Here's how the part is built. I have some questions about the finished solid (model axes, mm). A direction names the side the tool comes from. Coordinates: 2 decimals unless noted, no trailing zeros. Write each loop counter-clockwise with the first axis right and the second up, starting at its lowest first coordinate (ties: lowest second). Pieces come first, ordered by that corner, then holes.
from build123d import *

# Parameters (mm, degrees)
SKETCH3_R                   = 2.5
CUT_EXTRUDE1_DEPTH          = 10
CHAMFER1_SIZE               = 3
M8_TAPPED_HOLE1_D           = 6.8
M8_TAPPED_HOLE1_DEPTH       = 19.75
M8_TAPPED_HOLE1_CSINK_D     = 8.05
M8_TAPPED_HOLE1_CSINK_ANGLE = 90
M8_TAPPED_HOLE1_TIP         = 2.042926105


with BuildPart() as part:
    # Sketch1 → Revolve1 (revolve)
    with BuildSketch(Plane.XY, mode=Mode.PRIVATE) as revolve1_sk:
        Polygon((43, 0), (43, 10), (22.5, 10), (22.5, 20), (8.5, 20), (8.5, 9), (5, 9), (5, 3), (25, 3), (25, 0), align=None)
    revolve(revolve1_sk.sketch.rotate(Axis((0, 0, 0), (0, -1, 0)), 90), axis=Axis((0, 0, 0), (0, -1, 0)))

    # Sketch3 → Cut-Extrude1 (cut)
    with BuildSketch(Plane(origin=(0, 10, 0), x_dir=(1, 0, 0), z_dir=(0, 1, 0))):
        with Locations(Location((34, 0, 0), (0, 0, 270))):
            Circle(SKETCH3_R)
        with Locations(Location((0, -34, 0), (0, 0, 270))):
            Circle(SKETCH3_R)
        with Locations(Location((-34, 0, 0), (0, 0, 270))):
            Circle(SKETCH3_R)
        with Locations(Location((0, 34, 0), (0, 0, 270))):
            Circle(SKETCH3_R)
    extrude(amount=-CUT_EXTRUDE1_DEPTH, mode=Mode.SUBTRACT)

    # Chamfer1
    chamfer1_edges = [part.edges().sort_by_distance(p)[0] for p in [
        (0, 20, -22.5),
    ]]
    chamfer(chamfer1_edges, length=CHAMFER1_SIZE)

    # M8 Tapped Hole1
    with Locations(Plane(origin=(0, 10, -34), x_dir=(0, 0, 1), z_dir=(0, 1, 0))):
        with Locations((0, 0), (34, 34), (68, 0), (34, -34)):
            CounterSinkHole(M8_TAPPED_HOLE1_D / 2, M8_TAPPED_HOLE1_CSINK_D / 2, depth=M8_TAPPED_HOLE1_DEPTH, counter_sink_angle=M8_TAPPED_HOLE1_CSINK_ANGLE)
            with Locations((0, 0, -(M8_TAPPED_HOLE1_DEPTH + M8_TAPPED_HOLE1_TIP / 2))):  # 118° drill point
                Cone(0, M8_TAPPED_HOLE1_D / 2, M8_TAPPED_HOLE1_TIP, mode=Mode.SUBTRACT)


solid = part.part
1. Thinking about a two-plate mould opening in Z: for faces 1 (the face through (-5.901, 19.854, 18.738)), 2 (the face through (4, 9, 4)), 3 (the face through (19, 10, 19)), which applies, pulls with the +Z half, pulls with the -Z half, needs draft (parallel to the pull), parting line crosses it, or undercut?
2. I want a section at D-D (y = 13). List the corners of the cut face in (x, z) for me, then the cut area to 3 significant figures.
3. On a 3-axis mill with a long thin cutter (end or side, diameter ignored), from which of +Z, -Z, +X, -X, +Y, -Y can I reach the whole of each face in a straight line? I mean faces 4 (the face through (-8.428, 14.423, -1.107)), 5 (the face through (-1.3, 4.62, -37.14)), 6 (the face through (-7.509, 1.479, 23.846)). Say none if no direction works.
4. For pin 1 Ø2 at (x, z) = (-16, -15) entering from -Y; pin 2 Ø4 at (y, z) = (11, -17.5) entering from +X; pin 3 Ø22 at (x, z) = (0, 0) entering from +Y; pin 4 Ø8.5 at (x, z) = (-1, 3) entering from +Y, each with a flat end and sliding along its axis, tell me the tip position at first contact or that it passes through.
5. If I drill on line 1 (Y direction, x = -4, z = 35.5); line 2 (Z direction, x = -4, y = 3.5); line 3 (Y direction, x = 8.5, z = -7), over which ranges is the centre line in solid material (lowest first)?
6. I want a section at A-A (x = 0). State how many separate pieces and enclosed holes the cut face has, then the cut area to 3 significant figures.
7. I want a section at B-B (y = 6.5). List the corners of the cut face in (x, z) for me.
8. I want a section at C-C (x = 34). List the corners of the cut face in (y, z) for me (3 decimals).
Response values:
1. face 1: parting line crosses it
1. face 2: undercut
1. face 3: needs draft
2. outline: circle Ø45 at (0, 0); hole circle Ø17 at (0, 0)
2. area: 1,360 mm2
3. face 4: +Y
3. face 5: +Y, -Y
3. face 6: -Y
4. pin 1: stops at y = 3
4. pin 2: stops at x = 40
4. pin 3: stops at y = 20
4. pin 4: stops at y = 9
5. line 1: y = 0 to 10
5. line 2: z = -42.81 to -3, 3 to 42.81
5. line 3: y = 3 to 20
6. separate pieces: 4
6. enclosed holes: 0
6. area: 767 mm2
7. outline: circle Ø86 at (0, 0); hole circle Ø6.8 at (-34, 0); hole circle Ø10 at (0, 0); hole circle Ø6.8 at (0, -34); hole circle Ø6.8 at (0, 34); hole circle Ø6.8 at (34, 0)
8. outline: (0, -26.325) - (10, -26.325) - (10, -4.025) - (9.375, -3.4) - (0, -3.4) - close; (0, 3.4) - (9.375, 3.4) - (10, 4.025) - (10, 26.325) - (0, 26.325) - close
